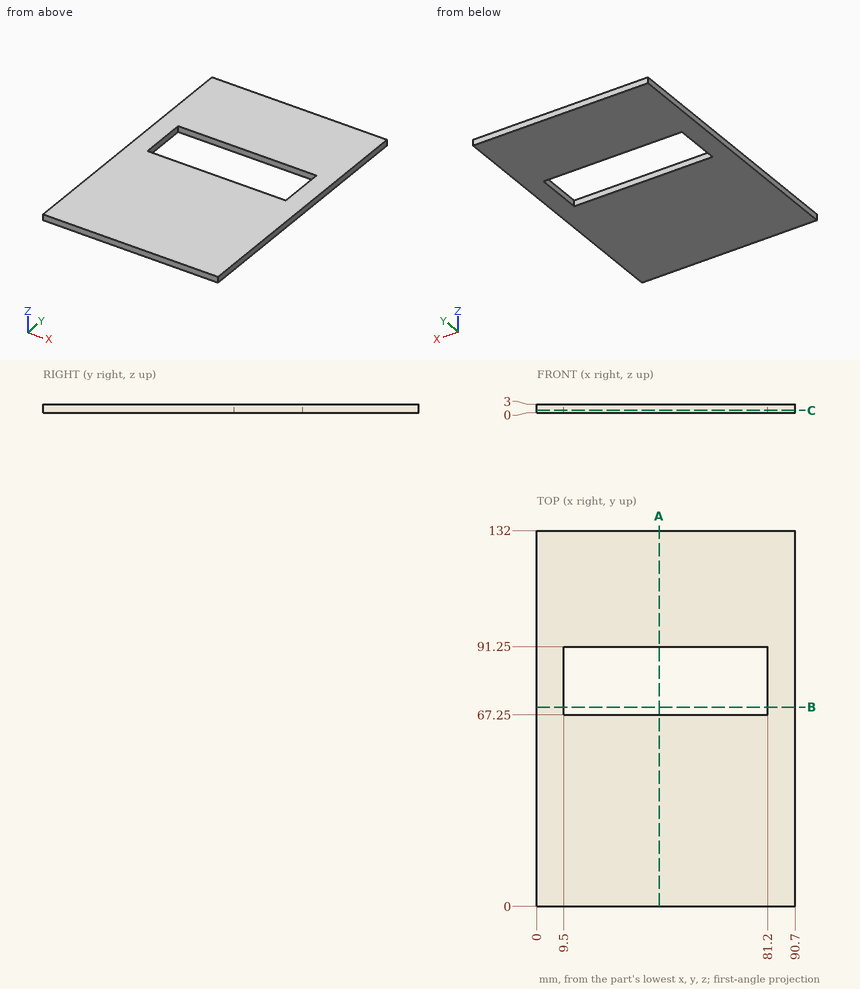
Part print with two shaded views. Sizes in mm from the minimum x, y, z corner. Round coordinates to 2 decimals unless told otherwise and drop trailing zeros. Write each loop counter-clockwise with the first axis right and the second up, starting at its lowest first coordinate (ties: lowest second). Pieces come first, ordered by that corner, then holes. Notation, with made-up numbers: M 51.25,26.25 L 99.25,26.25 A27 cw 99.25,58.25 Z; hole C 18.25,-16 d1. An arc over 180 degrees is marked long. Answer as CSV lines item,"result". Start each with the question number.
1) Drill centre lines: L1, parallel to Y at x = 27, z = 2.55; L2, parallel to X at y = 86, z = 1.15. Where is each one in solid material? Low to high.
2) Band-saw the part on A-A (x = 43). List the corners of the cut face in (y, z), then the cut area to 3 significant figures.
3) Band-saw the part on C-C (z = 0.8). List the corners of the cut face in (x, y).
4) Band-saw the part on B-B (y = 70). List the corners of the cut face in (x, z).
Worked out:
1,L1,"0 to 67.25, 91.25 to 132"
1,L2,"0 to 9.5, 81.2 to 90.7"
2,outline,"M 0,0 L 67.25,0 L 67.25,3 L 0,3 Z; M 91.25,0 L 132,0 L 132,3 L 91.25,3 Z"
2,area,"324 mm²"
3,outline,"M 0,0 L 90.7,0 L 90.7,132 L 0,132 Z; hole M 9.5,67.25 L 81.2,67.25 L 81.2,91.25 L 9.5,91.25 Z"
4,outline,"M 0,0 L 9.5,0 L 9.5,3 L 0,3 Z; M 81.2,0 L 90.7,0 L 90.7,3 L 81.2,3 Z"
